```python
from build123d import *

# Parameters (mm, degrees)
F1_DEPTH      = 15
F2_DEPTH      = 5
F2_DEPTH_BACK = 15
F3_DEPTH      = 15.001
F4_DEPTH      = 5


with BuildPart() as f1:
    # F0 (on Front) → F1 (new body)
    with BuildSketch(Plane.XZ):
        with BuildLine():
            ThreePointArc((0, 10), (6.123724, 7.905694), (9.682458, 2.5))
            Line((9.682458, 2.5), (20, 2.5))
            Line((20, 2.5), (20, 5))
            Line((20, 5), (15, 10))
            Line((15, 10), (0, 10))
        make_face()
        with BuildLine():
            ThreePointArc((4.330127, 2.5), (4.829629, 1.294095), (5, 0))
            ThreePointArc((5, 0), (4.829629, -1.294095), (4.330127, -2.5))
            Line((4.330127, -2.5), (9.682458, -2.5))
            Line((9.682458, -2.5), (20, -2.5))
            Line((20, -2.5), (20, 2.5))
            Line((20, 2.5), (9.682458, 2.5))
            Line((9.682458, 2.5), (4.330127, 2.5))
        make_face()
        with BuildLine():
            Line((20, -2.5), (9.682458, -2.5))
            ThreePointArc((9.682458, -2.5), (6.123724, -7.905694), (0, -10))
            Line((0, -10), (15, -10))
            Line((15, -10), (20, -5))
            Line((20, -5), (20, -2.5))
        make_face()
        with BuildLine():
            ThreePointArc((4.330127, -2.5), (4.829629, -1.294095), (5, 0))
            ThreePointArc((5, 0), (4.829629, 1.294095), (4.330127, 2.5))
            ThreePointArc((4.330127, 2.5), (0, 5), (-4.330127, 2.5))
            ThreePointArc((-4.330127, 2.5), (-5, 0), (-4.330127, -2.5))
            ThreePointArc((-4.330127, -2.5), (0, -5), (4.330127, -2.5))
        make_face()
        with BuildLine():
            ThreePointArc((-4.330127, -2.5), (-5, 0), (-4.330127, 2.5))
            Line((-4.330127, 2.5), (-9.682458, 2.5))
            ThreePointArc((-9.682458, 2.5), (-10, 0), (-9.682458, -2.5))
            Line((-9.682458, -2.5), (-4.330127, -2.5))
        make_face()
    extrude(amount=-F1_DEPTH)

    # F0 (on Front) → F2 (join, two sides)
    with BuildSketch(Plane.XZ) as f2_sk:
        with BuildLine():
            ThreePointArc((-4.330127, 2.5), (0, 5), (4.330127, 2.5))
            Line((4.330127, 2.5), (9.682458, 2.5))
            ThreePointArc((9.682458, 2.5), (6.123724, 7.905694), (0, 10))
            ThreePointArc((0, 10), (-6.123724, 7.905694), (-9.682458, 2.5))
            Line((-9.682458, 2.5), (-4.330127, 2.5))
        make_face()
        with BuildLine():
            Line((9.682458, -2.5), (4.330127, -2.5))
            ThreePointArc((4.330127, -2.5), (0, -5), (-4.330127, -2.5))
            Line((-4.330127, -2.5), (-9.682458, -2.5))
            ThreePointArc((-9.682458, -2.5), (-6.123724, -7.905694), (0, -10))
            ThreePointArc((0, -10), (6.123724, -7.905694), (9.682458, -2.5))
        make_face()
    extrude(amount=F2_DEPTH)
    extrude(f2_sk.sketch, amount=-F2_DEPTH_BACK)

    # F0 (on Front) → F3 (cut, through all)
    with BuildSketch(Plane.XZ):
        with BuildLine():
            ThreePointArc((4.330127, -2.5), (4.829629, -1.294095), (5, 0))
            ThreePointArc((5, 0), (4.829629, 1.294095), (4.330127, 2.5))
            ThreePointArc((4.330127, 2.5), (0, 5), (-4.330127, 2.5))
            ThreePointArc((-4.330127, 2.5), (-5, 0), (-4.330127, -2.5))
            ThreePointArc((-4.330127, -2.5), (0, -5), (4.330127, -2.5))
        make_face()
    extrude(amount=-F3_DEPTH, mode=Mode.SUBTRACT)

    # F0 (on Front) → F4 (cut)
    with BuildSketch(Plane.XZ):
        with BuildLine():
            ThreePointArc((4.330127, 2.5), (4.829629, 1.294095), (5, 0))
            ThreePointArc((5, 0), (4.829629, -1.294095), (4.330127, -2.5))
            Line((4.330127, -2.5), (9.682458, -2.5))
            Line((9.682458, -2.5), (20, -2.5))
            Line((20, -2.5), (20, 2.5))
            Line((20, 2.5), (9.682458, 2.5))
            Line((9.682458, 2.5), (4.330127, 2.5))
        make_face()
        with BuildLine():
            ThreePointArc((-4.330127, -2.5), (-5, 0), (-4.330127, 2.5))
            Line((-4.330127, 2.5), (-9.682458, 2.5))
            ThreePointArc((-9.682458, 2.5), (-10, 0), (-9.682458, -2.5))
            Line((-9.682458, -2.5), (-4.330127, -2.5))
        make_face()
    extrude(amount=-F4_DEPTH, mode=Mode.SUBTRACT)


solid = f1.part
```
The listing builds one solid part. Answer for the finished solid, in the listing's coordinates (mm). A direction names the side the tool comes from. Coordinates: 2 decimals unless noted, no trailing zeros. Write each loop counter-clockwise with the first axis right and the second up, starting at its lowest first coordinate (ties: lowest second). Pieces come first, ordered by that corner, then holes. Notation, with made-up numbers: (33.25, 70.5) - (92.25, 70.5) arc R22 ccw to (92.25, 80.5) - close; hole circle Ø5 at (9, -9). An arc over 180 degrees is marked (long way). Return JSON: item names as keys, results as strings. Group by question number.
1. Which of the six approach directions +Z, -Z, +X, -X, +Y, -Y give full straight-line access (tool end or side, diameter ignored) to faces 1 (the flat face through (12, 0, -6)), 2 (the cylindrical face through (-10, 10, 0)), 3 (the flat face through (12, 5, 0))?
2. Given pin 1 (6 mm diameter, centred on x = -7, y = -1.5, fed in from +Z); pin 2 (10 mm diameter, centred on x = -2, y = 7, fed in from +Z); pin 3 (8 mm diameter, centred on y = 2, z = -7.5, fed in from -X); pin 4 (1.5 mm diameter, centred on y = 12, z = -1, fed in from -X), each flat-ended and moving along its own axis, determine where each tip first touches the part or whether it passes through.
3. A cutting plane is placed at C-C, the plane y = 13.75. Determine the outline of the cut face in (x, z), plus the area to 3 significant figures.
4. Straight lines are drawn through the part: L1, parallel to Z at x = 9, y = 1.5; L2, parallel to Z at x = 2.5, y = 6.5; L3, parallel to Y at x = 12.75, z = 8.75. For each, find the intervals that lie inside material, in ascending order.
5. A cutting plane is placed at D-D, the plane z = -4.5. Determine the outline of the cut face in (x, y).
6. A cutting plane is placed at A-A, the plane y = 2.75. Determine the outline of the cut face in (x, z), plus the area to 3 significant figures.
7. Determine the mould class of faces 4 (the flat face through (10, 1, -2.5)), 5 (the flat face through (12, 0, 6)), 6 (the flat face through (8, 7, 10)) for opening direction Z: released by +Z, released by -Z, zero draft, split by the parting line, or undercut.
Ans:
{
 "1": {"face 1": "-Z, +X, -Y", "face 2": "-X, +Y, -Y", "face 3": "+X, -X, -Y"},
 "2": {"pin 1": "z = 9.17", "pin 2": "z = 10", "pin 3": "x = -9.37", "pin 4": "x = -10"},
 "3": {"outline": "(-9.68, -2.5) arc R10 ccw to (0, -10) - (15, -10) - (20, -5) - (20, 5) - (15, 10) - (0, 10) arc R10 ccw to (-9.68, 2.5) arc R10 ccw to start; hole (4.33, -2.5) arc R5 ccw to (5, 0) arc R5 ccw to (4.33, 2.5) arc R5 ccw (long way) to start", "area": "454 mm²"},
 "4": {"L1": "-10 to -2.5, 2.5 to 10", "L2": "-10 to -4.33, 4.33 to 10", "L3": "0 to 15"},
 "5": {"outline": "(-8.93, -5) - (-2.18, -5) - (-2.18, 15) - (-8.93, 15) - close; (2.18, -5) - (8.93, -5) - (8.93, 0) - (20, 0) - (20, 15) - (2.18, 15) - close"},
 "6": {"outline": "(-9.68, -2.5) arc R10 ccw to (0, -10) - (15, -10) - (20, -5) - (20, -2.5) - (4.33, -2.5) arc R5 cw to (-4.33, -2.5) - close; (-9.68, 2.5) - (-4.33, 2.5) arc R5 cw to (4.33, 2.5) - (20, 2.5) - (20, 5) - (15, 10) - (0, 10) arc R10 ccw to start", "area": "352 mm²"},
 "7": {"face 4": "undercut", "face 5": "zero draft", "face 6": "released by +Z"}
}
